Here's how the part is built. I have some questions about the finished solid (model axes, mm). A direction names the side the tool comes from. Coordinates: 2 decimals unless noted, no trailing zeros. Write each loop counter-clockwise with the first axis right and the second up, starting at its lowest first coordinate (ties: lowest second). Pieces come first, ordered by that corner, then holes.
(1) Imagine slicing it at B-B, the plane y = 5. List the corners of the cut face in (x, z) for me.
(2) Imagine slicing it at A-A, the plane x = -4.75. List the corners of the cut face in (y, z) for me, plus the area to 3 significant figures.
(3) Imagine slicing it at D-D, the plane y = 2.25. List the corners of the cut face in (x, z) for me, plus the area to 3 significant figures.
(4) For pin 1 Ø5 at (x, y) = (44.5, 8) entering from +Z; pin 2 Ø5 at (y, z) = (5.5, 7.5) entering from -X; pin 3 Ø3.5 at (x, y) = (44.75, 15) entering from -Z; pin 4 Ø2.5 at (x, y) = (-4.75, 5) entering from +Z, each with a flat end and sliding along its axis, tell me the tip position at first contact or that it passes through.
(5) Thinking about a two-plate mould opening in Y: for faces 5 (the cylindrical face through (7.474, 8.648, 46.479)), 6 (the flat face through (20, 20, 22)), 7 (the cylindrical face through (-3.25, 14.95, 38.01)), which applies, released by +Y, released by -Y, zero draft, split by the parting line, or undercut?
(6) Please list where these lines run through material, in increasing order: probe 1 along Y at (x, z) = (44.75, 38); probe 2 along Z at (x, y) = (18.5, 14); probe 3 along Z at (x, y) = (43, 19).
(7) Imagine slicing it at C-C, the plane z = 21. List the corners of the cut face in (x, y) for me.
(8) Which directions (+Z, -Z, +X, -X, +Y, -Y) give clear straight access to the entire face, cutting with the end or side of a thin tool? Please do faces 1 (the flat face through (43, 10, 37)), 2 (the flat face through (-3, 10, 37)), 3 (the flat face through (-3, 10, 39)), 4 (the flat face through (40, 10, 42)).
```python
from build123d import *

# Parameters (mm, degrees)
ESQUISSE1_W             = 40
ESQUISSE1_H             = 20
BOSS_EXTRU_1_DEPTH      = 45
ESQUISSE2_R             = 2
BOSS_EXTRU_2_DEPTH      = 3
ESQUISSE3_W             = 2
ESQUISSE3_H             = 20
BOSS_EXTRU_3_DEPTH      = 6
ESQUISSE4_W             = 2
ESQUISSE4_H             = 20
BOSS_EXTRU_4_DEPTH      = 6
ESQUISSE5_R             = 1.5
ENL_V_MAT_EXTRU_1_DEPTH = 6


with BuildPart() as part:
    # Esquisse1 → Boss.-Extru.1 (new body)
    with BuildSketch(Plane.XY):
        with Locations((20, 10)):
            Rectangle(ESQUISSE1_W, ESQUISSE1_H)
    extrude(amount=BOSS_EXTRU_1_DEPTH)

    # Esquisse2 → Boss.-Extru.2 (add)
    with BuildSketch(Plane.XY.offset(45)):
        with Locations(Location((6, 10, 0), (0, 0, 180))):
            Circle(ESQUISSE2_R)
    extrude(amount=BOSS_EXTRU_2_DEPTH)

    # Esquisse3 → Boss.-Extru.3 (add)
    with BuildSketch(Plane.ZY):
        with Locations((38, 10)):
            Rectangle(ESQUISSE3_W, ESQUISSE3_H)
    extrude(amount=BOSS_EXTRU_3_DEPTH)

    # Esquisse4 → Boss.-Extru.4 (add)
    with BuildSketch(Plane(origin=(40, 0, 0), x_dir=(0, 0, -1), z_dir=(1, 0, 0))):
        with Locations((-38, 10)):
            Rectangle(ESQUISSE4_W, ESQUISSE4_H)
    extrude(amount=BOSS_EXTRU_4_DEPTH)

    # Esquisse5 → Enlèv. mat.-Extru.1 (cut)
    with BuildSketch(Plane.XY.offset(39)):
        with Locations((-4.75, 15)):
            Circle(ESQUISSE5_R)
        with Locations((44.75, 15)):
            Circle(ESQUISSE5_R)
        with Locations((44.75, 5)):
            Circle(ESQUISSE5_R)
        with Locations((-4.75, 5)):
            Circle(ESQUISSE5_R)
    extrude(amount=-ENL_V_MAT_EXTRU_1_DEPTH, mode=Mode.SUBTRACT)


solid = part.part
```
Recorded:
1. outline: (-3.25, 37) - (0, 37) - (0, 0) - (40, 0) - (40, 37) - (43.25, 37) - (43.25, 39) - (40, 39) - (40, 45) - (0, 45) - (0, 39) - (-3.25, 39) - close
2. outline: (0, 37) - (3.5, 37) - (3.5, 39) - (0, 39) - close; (6.5, 37) - (13.5, 37) - (13.5, 39) - (6.5, 39) - close; (16.5, 37) - (20, 37) - (20, 39) - (16.5, 39) - close
2. area: 28.0 mm2
3. outline: (-6, 37) - (0, 37) - (0, 0) - (40, 0) - (40, 37) - (46, 37) - (46, 39) - (40, 39) - (40, 45) - (0, 45) - (0, 39) - (-6, 39) - close
3. area: 1,820 mm2
4. pin 1: stops at z = 39
4. pin 2: stops at x = 0
4. pin 3: stops at z = 37
4. pin 4: passes through
5. face 5: split by the parting line
5. face 6: released by +Y
5. face 7: undercut
6. probe 1: y = 0 to 3.5, 6.5 to 13.5, 16.5 to 20
6. probe 2: z = 0 to 45
6. probe 3: z = 37 to 39
7. outline: (0, 0) - (40, 0) - (40, 20) - (0, 20) - close
8. face 1: -Z, +X, +Y, -Y
8. face 2: -Z, -X, +Y, -Y
8. face 3: +Z, -X, +Y, -Y
8. face 4: +Z, +X, +Y, -Y
